```python
from build123d import *

# Parameters (mm, degrees)
SKETCH2_R           = 41.75
SKETCH2_R_2         = 41.25
BOSS_EXTRUDE1_DEPTH = 28
BOSS_EXTRUDE2_START = -2
SKETCH2_3_R         = 41.75
SKETCH2_3_R_2       = 2
SKETCH2_3_R_3       = 1.5
SKETCH2_3_R_4       = 32.5
BOSS_EXTRUDE2_DEPTH = 2


with BuildPart() as part:
    # Sketch2 → Boss-Extrude1 (new body)
    with BuildSketch(Plane.XY):
        with Locations(Location((-114.563267105, -12.719508093, 0), (0, 0, 180))):
            Circle(SKETCH2_R)
        with Locations(Location((-114.563267105, -12.719508093, 0), (0, 0, 180))):
            Circle(SKETCH2_R_2, mode=Mode.SUBTRACT)
    extrude(amount=BOSS_EXTRUDE1_DEPTH)

    # Sketch2<3> → Boss-Extrude2 (add)
    with BuildSketch(Plane.XY.offset(BOSS_EXTRUDE2_START)):
        with Locations(Location((-114.563267105, -12.719508093, 0), (0, 0, 180))):
            Circle(SKETCH2_3_R)
        with Locations((-143.38415281, -35.116082543)):
            Circle(SKETCH2_3_R_2, mode=Mode.SUBTRACT)
        with Locations((-122.245105889, -48.401987728)):
            Circle(SKETCH2_3_R_2, mode=Mode.SUBTRACT)
        with Locations((-149.30612033, -23.908080375)):
            Circle(SKETCH2_3_R_3, mode=Mode.SUBTRACT)
        with Locations((-97.511641226, -44.991664124)):
            Circle(SKETCH2_3_R_2, mode=Mode.SUBTRACT)
        with Locations((-87.502252663, -37.213415445)):
            Circle(SKETCH2_3_R_3, mode=Mode.SUBTRACT)
        with Locations((-80.756821819, -26.480840048)):
            Circle(SKETCH2_3_R_2, mode=Mode.SUBTRACT)
        with Locations((-151.037587002, -11.350571264)):
            Circle(SKETCH2_3_R_2, mode=Mode.SUBTRACT)
        with Locations((-141.624281546, 11.77439926)):
            Circle(SKETCH2_3_R_2, mode=Mode.SUBTRACT)
        with Locations((-119.548826684, 23.438398314)):
            Circle(SKETCH2_3_R_2, mode=Mode.SUBTRACT)
        with Locations((-114.563267105, -12.719508093)):
            Circle(SKETCH2_3_R_4, mode=Mode.SUBTRACT)
        with Locations((-79.820413879, -1.53093581)):
            Circle(SKETCH2_3_R_2, mode=Mode.SUBTRACT)
        with Locations((-95.140573086, 18.183711109)):
            Circle(SKETCH2_3_R_2, mode=Mode.SUBTRACT)
        with Locations((-106.88142832, 22.962971542)):
            Circle(SKETCH2_3_R_3, mode=Mode.SUBTRACT)
    extrude(amount=BOSS_EXTRUDE2_DEPTH)


solid = part.part
```
CAD build for the part. Positions are in the model's coordinates, mm. A direction names the side the tool comes from. Round coordinates to 2 decimals unless told otherwise and drop trailing zeros. Order: outer loops, then holes, each group sorted by start corner. A loop starts at its lowest first (then second) coordinate and runs counter-clockwise, first axis right, second up. Notation, with made-up numbers: (67, -30) -> (108, -30) arc R20 cw to (108, -7) -> close; hole circle Ø1 at (63, 67). An arc over 180 degrees is marked (long way). Write item = value, one per line.
(1) Cut at B-B (y = -29.5). Write the cut outline in (x, z).
Answers follow:
outline = (-152.79, -2) -> (-142.4, -2) -> (-142.4, 0) -> (-152.25, 0) -> (-152.25, 28) -> (-152.79, 28) -> close; (-86.73, -2) -> (-76.33, -2) -> (-76.33, 28) -> (-76.88, 28) -> (-76.88, 0) -> (-86.73, 0) -> close
(2) Cut at C-C (y = -44). Write the cut outline in (x, z), plus the area to 3 significant figures.
Answers follow:
outline = (-142.21, -2) -> (-123.38, -2) -> (-123.38, 0) -> (-141.45, 0) -> (-141.45, 28) -> (-142.21, 28) -> close; (-105.74, -2) -> (-99.25, -2) -> (-99.25, 0) -> (-105.74, 0) -> close; (-95.77, -2) -> (-86.91, -2) -> (-86.91, 28) -> (-87.67, 28) -> (-87.67, 0) -> (-95.77, 0) -> close
area = 111 mm²
(3) 3-axis set-ups, long thin cutter, end or side, ignore diameter. For faces 1 (the flat face through (-84, -25, 0)), 2 (the cylindrical face through (-78.85, -25.88, -1.01)): which of +Z, -Z, +X, -X, +Y, -Y reach the whole face in a straight line?
Answers follow:
face_1 = +Z
face_2 = +Z, -Z
(4) Cut at A-A (x = -135.5). Write the cut outline in (y, z), plus the area to 3 significant figures.
Answers follow:
outline = (-48.84, -2) -> (-37.58, -2) -> (-37.58, 0) -> (-48.26, 0) -> (-48.26, 28) -> (-48.84, 28) -> close; (12.14, -2) -> (23.4, -2) -> (23.4, 28) -> (22.82, 28) -> (22.82, 0) -> (12.14, 0) -> close
area = 77.5 mm²
(5) Pull direction X, two halves, no side cores. Call faces 3 (the flat face through (-105, -53, 28)), 4 (the cylindrical face through (-141.537, -35.882, -1.014)), 5 (the cylindrical face through (-153.13, 3.27, 12.79)), 6 (the cylindrical face through (-147.03, -11.29, -1.01)): +X half, -X half, draft (parallel to the pull), parting line (faces both ways), or undercut.
Answers follow:
face_3 = draft
face_4 = undercut
face_5 = parting line
face_6 = undercut
(6) Cut at D-D (z = 2.25). Write the cut outline in (x, y), plus the area to 3 significant figures.
Answers follow:
outline = circle Ø83.5 at (-114.56, -12.72); hole circle Ø82.5 at (-114.56, -12.72)
area = 130 mm²
(7) Drill centre lines: L1, parallel to X at y = -17, z = 6.75; L2, parallel to X at y = -28, z = 2.5; L3, parallel to Y at x = -136.5, z = 23.5. Where is each one in solid material? Low to high.
Answers follow:
L1 = -156.09 to -155.59, -73.54 to -73.03
L2 = -153.42 to -152.88, -76.25 to -75.71
L3 = -48.24 to -47.65, 22.21 to 22.8
(8) Flat gauge pins, fed straight in: P1, Ø4, axis at x = -105, z = 15.5, coming from the +Y side; P2, Ø10, axis at y = -25.5, z = 5, coming from the -X side; P3, Ø10, axis at x = -113.5, z = 15, coming from the -Y side. Where does each tip first touch, or does it go through?
Answers follow:
P1 = 28.34
P2 = -155.58
P3 = -54.47
